Verification items for the finished model (mm, model axes). A direction names the side the tool comes from. Coordinates: 2 decimals unless noted, no trailing zeros. Order: outer loops, then holes, each group sorted by start corner. A loop starts at its lowest first (then second) coordinate and runs counter-clockwise, first axis right, second up. Notation, with made-up numbers: (2, 56) -> (36, 56) arc R19 cw to (36, 92) -> close; hole circle Ø5 at (82, -18.75). An arc over 180 degrees is marked (long way). Write item = value, one per line. Start each with the question number.
1. Cross-section at A-A on y = 15. Record the cut outline in (x, z).
2. Release check for a two-part mould opening along X. For faces 6 (the cylindrical face through (28.17, -16.93, 7.4)), 7 (the cylindrical face through (1.08, 19.88, 32.61)), 8 (the flat face through (21.357, -40.66, 2.535)), 9 (the flat face through (-1, 0, 20)) record: +X half, -X half, draft (parallel to the pull), parting line (faces both ways), or undercut.
3. Cross-section at C-C on x = -30.5. Record the cut outline in (y, z), plus the area to 3 significant figures.
4. Set-up check for faces 1 (the flat face through (-40, -10, 20)), 2 (the flat face through (32.046, -116.977, 37.535)), 3 (the flat face through (7, -88, 5)), 4 (the flat face through (-36.465, -18, 20)), 5 (the cylindrical face through (-28.35, -14.65, 7.4)): record each of +Z, -Z, +X, -X, +Y, -Y from which the full face is reachable in a straight line by a thin tool's end or side.
5. Thickness scan on line 1 along X through (y, z) = (15, 11); line 2 along Z through (x, y) = (23, -134.5); line 3 along Y through (x, z) = (35, 11.5). Record the ranges inside material, lowest first. Write a range as from..to.
6. Go/stop test with flat-tipped pins: P1, Ø5, axis at x = -20, y = -29, coming from the -Z side; P2, Ø1.4, axis at y = -18.5, z = 20, coming from the +X side; P3, Ø8, axis at x = -16, z = 6.5, coming from the -Y side; P4, Ø12, axis at x = -26, z = 11, coming from the -Y side. Record where each tip stops, or that it passes through.
7. Cross-section at B-B on y = -109. Record the cut outline in (x, z), plus the area to 3 significant figures.
8. Cross-section at D-D on z = 10. Record the cut outline in (x, y) (3 decimals), plus the area to 3 significant figures.
from build123d import *

# Parameters (mm, degrees)
SALIENTE_EXTRUIR1_DEPTH    = 40
CROQUIS2_R                 = 5
SALIENTE_EXTRUIR2_DEPTH    = 5
SALIENTE_EXTRUIR3_START    = -35
CROQUIS2_4_R               = 5
SALIENTE_EXTRUIR3_DEPTH    = 5
CORTAR_EXTRUIR1_DEPTH      = 167.172965861
REDONDEO5_R                = 2
CORTAR_EXTRUIR2_DEPTH      = 5
CORTAR_EXTRUIR3_DEPTH      = 164.7261433
CORTAR_EXTRUIR3_DEPTH_BACK = 164.7261433
CROQUIS4_4_R               = 2.5
SALIENTE_EXTRUIR5_START    = 20
CROQUIS7_R                 = 20
CROQUIS7_R_2               = 5
SALIENTE_EXTRUIR5_DEPTH    = 15
SALIENTE_EXTRUIR6_START    = -5
CROQUIS7_2_R               = 20
CROQUIS7_2_R_2             = 5
SALIENTE_EXTRUIR6_DEPTH    = 15


with BuildPart() as part:
    # Croquis1 → Saliente-Extruir1 (new body)
    with BuildSketch(Plane.XY):
        with BuildLine():
            Line((-37, 0), (37, 0))
            ThreePointArc((37, 0), (39.121320344, -0.878679656), (40, -3))
            Line((40, -3), (40, -17))
            ThreePointArc((40, -17), (39.121320344, -19.121320344), (37, -20))
            Line((37, -20), (-37, -20))
            ThreePointArc((-37, -20), (-39.121320344, -19.121320344), (-40, -17))
            Line((-40, -17), (-40, -3))
            ThreePointArc((-40, -3), (-39.121320344, -0.878679656), (-37, 0))
        make_face()
    extrude(amount=SALIENTE_EXTRUIR1_DEPTH)

    # Croquis2 → Saliente-Extruir2 (add)
    with BuildSketch(Plane.XY.offset(40)):
        with BuildLine():
            Line((-25, -20), (0.692322562, -77.955122319))
            Line((0.692322562, -77.955122319), (5.041226188, -141.200506964))
            ThreePointArc((5.041226188, -141.200506964), (26.438391415, -157.05107249), (38.716761316, -133.422260844))
            Line((38.716761316, -133.422260844), (25.186319846, -100.064303858))
            Line((25.186319846, -100.064303858), (17.814778444, -60.749416381))
            Line((17.814778444, -60.749416381), (25, -20))
            Line((25, -20), (0, -20))
            Line((0, -20), (-25, -20))
        make_face()
        with Locations((22.5, -140)):
            Circle(CROQUIS2_R, mode=Mode.SUBTRACT)
    extrude(amount=-SALIENTE_EXTRUIR2_DEPTH)

    # Croquis2<4> → Saliente-Extruir3 (add)
    with BuildSketch(Plane.XY.offset(40).offset(SALIENTE_EXTRUIR3_START)):
        with BuildLine():
            Line((-25, -20), (0.692322562, -77.955122319))
            Line((0.692322562, -77.955122319), (5.041226188, -141.200506964))
            ThreePointArc((5.041226188, -141.200506964), (26.438391415, -157.05107249), (38.716761316, -133.422260844))
            Line((38.716761316, -133.422260844), (25.186319846, -100.064303858))
            Line((25.186319846, -100.064303858), (17.814778444, -60.749416381))
            Line((17.814778444, -60.749416381), (25, -20))
            Line((25, -20), (0, -20))
            Line((0, -20), (-25, -20))
        make_face()
        with Locations((22.5, -140)):
            Circle(CROQUIS2_4_R, mode=Mode.SUBTRACT)
    extrude(amount=-SALIENTE_EXTRUIR3_DEPTH)

    # Croquis3 → Cortar-Extruir1 (cut, through all)
    with BuildSketch(Plane(origin=(0, -1.419488972, 40.648845743), x_dir=(1, 0, 0), z_dir=(0, -0.034899496702501046, 0.9993908270190958))):
        Polygon((-19.530157581, -18.591836672), (19.922773595, -18.591836672), (12.964371873, -58.030854026), (-2.035628127, -58.030854026), align=None)
    extrude(amount=CORTAR_EXTRUIR1_DEPTH, mode=Mode.SUBTRACT)

    # Redondeo5
    # the kernel refuses this fillet: 2 mm, written as the material it adds along each edge
    with BuildSketch(Plane(origin=(17.715799962, -59.41499217, 38.623598144), x_dir=(0, 0.9993908270190957, 0.03489949670250261), z_dir=(-1, 0, 0))) as redondeo5_piece_1:
        with BuildLine():
            CenterArc((1.900571235, -2), REDONDEO5_R, 90, 71.857609754)
            Line((0, -1.377240834), (-0.038011425, -1.364785651))
            ThreePointArc((-0.038011425, -1.364785651), (-0.04, -0.688620417), (-0.04, 0))
            Line((-0.04, 0), (0, 0.04))
            Line((0, 0.04), (1.900571235, 0.04))
            Line((1.900571235, 0.04), (1.900571235, 0))
        make_face()
    extrude(amount=24.502856177)

    # Croquis4 → Cortar-Extruir2 (cut, symmetric)
    with BuildSketch(Plane.XY.offset(20)):
        with BuildLine():
            Line((-36.464835441, -15.405002376), (-36.464835441, -20))
            Line((-36.464835441, -20), (-25, -20))
            Line((-25, -20), (-25, -15.405002376))
            ThreePointArc((-25, -15.405002376), (-30.732417721, -9.672584656), (-36.464835441, -15.405002376))
        make_face()
        with BuildLine():
            Line((36.338744123, -15.405012958), (36.338744123, -20))
            Line((36.338744123, -20), (23.961776552, -20))
            Line((23.961776552, -20), (23.961776552, -15.405012958))
            ThreePointArc((23.961776552, -15.405012958), (30.150260338, -9.216529173), (36.338744123, -15.405012958))
        make_face()
    extrude(amount=CORTAR_EXTRUIR2_DEPTH, both=True, mode=Mode.SUBTRACT)

    # Croquis4<4> → Cortar-Extruir3 (cut, two sides: drawn at the far end of the back side and taken through both)
    with BuildSketch(Plane.XY.offset(20).offset(-CORTAR_EXTRUIR3_DEPTH_BACK)):
        with Locations((-30.732417721, -15.405002376)):
            Circle(CROQUIS4_4_R)
        with Locations((30.150260338, -15.405012958)):
            Circle(CROQUIS4_4_R)
    extrude(amount=CORTAR_EXTRUIR3_DEPTH + CORTAR_EXTRUIR3_DEPTH_BACK, mode=Mode.SUBTRACT)

    # Croquis7 → Saliente-Extruir5 (add)
    with BuildSketch(Plane.XY.offset(20).offset(SALIENTE_EXTRUIR5_START)):
        with Locations((0, 15)):
            Circle(CROQUIS7_R)
        with Locations(Location((0, 15, 0), (0, 0, 180))):
            Circle(CROQUIS7_R_2, mode=Mode.SUBTRACT)
    extrude(amount=-SALIENTE_EXTRUIR5_DEPTH)

    # Croquis7<2> → Saliente-Extruir6 (add)
    with BuildSketch(Plane.XY.offset(20).offset(SALIENTE_EXTRUIR6_START)):
        with Locations((0, 15)):
            Circle(CROQUIS7_2_R)
        with Locations(Location((0, 15, 0), (0, 0, 180))):
            Circle(CROQUIS7_2_R_2, mode=Mode.SUBTRACT)
    extrude(amount=-SALIENTE_EXTRUIR6_DEPTH)


solid = part.part
Worked out:
q1.outline = (-20, 0) -> (-5, 0) -> (-5, 15) -> (-20, 15) -> close; (-20, 25) -> (-5, 25) -> (-5, 40) -> (-20, 40) -> close; (5, 0) -> (20, 0) -> (20, 15) -> (5, 15) -> close; (5, 25) -> (20, 25) -> (20, 40) -> (5, 40) -> close
q2.face_6 = undercut
q2.face_7 = undercut
q2.face_8 = +X half
q2.face_9 = draft
q3.outline = (-20, 0) -> (-17.89, 0) -> (-17.89, 15) -> (-20, 15) -> close; (-20, 25) -> (-17.89, 25) -> (-17.89, 40) -> (-20, 40) -> close; (-12.92, 0) -> (0, 0) -> (0, 40) -> (-12.92, 40) -> (-12.92, 25) -> (-9.68, 25) -> (-9.68, 15) -> (-12.92, 15) -> close
q3.area = 547 mm²
q4.face_1 = +Z, -Z, -X, +Y, -Y
q4.face_2 = +Z, -Z, +X
q4.face_3 = +X, -X, -Y
q4.face_4 = -Y
q4.face_5 = +Z, -Z
q5.line_1 = -20..-5, 5..20
q5.line_2 = 0..5, 35..40
q5.line_3 = -20..0
q6.P1 = 0
q6.P2 = 39.89
q6.P3 = -48.67
q6.P4 = -20
q7.outline = (2.83, 0) -> (28.81, 0) -> (28.81, 5) -> (2.83, 5) -> close; (2.83, 35) -> (28.81, 35) -> (28.81, 40) -> (2.83, 40) -> close
q7.area = 260 mm²
q8.outline = (-40, -17) arc R3 ccw to (-37, -20) -> (37, -20) arc R3 ccw to (40, -17) -> (40, -3) arc R3 ccw to (37, 0) -> (13.229, 0) arc R20 ccw (long way) to (-13.229, 0) -> (-37, 0) arc R3 ccw to (-40, -3) -> close; hole circle Ø5 at (-30.732, -15.405); hole circle Ø10 at (0, 15); hole circle Ø5 at (30.15, -15.405)
q8.area = 2,640 mm²
